```python
from build123d import *

# Parameters (mm, degrees)
SKETCH1_W           = 40
SKETCH1_H           = 40
BOSS_EXTRUDE1_DEPTH = 3
SKETCH3_W           = 20
SKETCH3_H           = 3
EXTRUDE_THIN1_DEPTH = 20
SKETCH4_W           = 10
SKETCH4_H           = 17
BOSS_EXTRUDE2_DEPTH = 2
EXTRUDE_THIN2_DEPTH = 20
SKETCH6_R           = 12.5
CUT_EXTRUDE1_DEPTH  = 57.789083458
SKETCH7_R           = 1.75
CUT_EXTRUDE2_DEPTH  = 55.990908339
CIRPATTERN1_COUNT   = 5
SKETCH8_R           = 1.75
CUT_EXTRUDE3_DEPTH  = 10
SKETCH9_R           = 1.75
CUT_EXTRUDE4_DEPTH  = 10
CUT_EXTRUDE5_DEPTH  = 59.72818744
FILLET1_R           = 2
FILLET3_R           = 2
FILLET4_R           = 2
FILLET5_R           = 2
FILLET2_R           = 1


with BuildPart() as part:
    # Sketch1 → Boss-Extrude1 (new body)
    with BuildSketch(Plane.XY):
        with Locations((0, 20)):
            Rectangle(SKETCH1_W, SKETCH1_H)
    extrude(amount=-BOSS_EXTRUDE1_DEPTH)

    # Sketch3 → Extrude-Thin1 (add, symmetric)
    with BuildSketch(Plane(origin=(0, 0, 0), x_dir=(0, 0, -1), z_dir=(1, 0, 0))):
        with Locations((-7, -1.5)):
            Rectangle(SKETCH3_W, SKETCH3_H)
    extrude(amount=EXTRUDE_THIN1_DEPTH, both=True)

    # Sketch4 → Boss-Extrude2 (add)
    with BuildSketch(Plane(origin=(0, 0, 0), x_dir=(1, 0, 0), z_dir=(0, 1, 0))):
        with Locations((0, -8.5)):
            Rectangle(SKETCH4_W, SKETCH4_H)
    extrude(amount=BOSS_EXTRUDE2_DEPTH)

    # Sketch5 → Extrude-Thin2 (add, symmetric)
    with BuildSketch(Plane(origin=(0, 0, 0), x_dir=(0, 0, -1), z_dir=(1, 0, 0))):
        Polygon((-17, 17), (-17, -8), (-32, -8), (-32, -3), (-29, -3), (-29, -5), (-20, -5), (-20, 17), align=None)
    extrude(amount=EXTRUDE_THIN2_DEPTH, both=True)

    # Sketch6 → Cut-Extrude1 (cut, through all)
    with BuildSketch(Plane.XY.offset(32)):
        with Locations((0, 20)):
            Circle(SKETCH6_R)
    extrude(amount=-CUT_EXTRUDE1_DEPTH, mode=Mode.SUBTRACT)

    # Sketch7 → Cut-Extrude2 (cut, through all)
    with BuildSketch(Plane.XY):
        with Locations((0, 37.5)):
            Circle(SKETCH7_R)
    cut_extrude2 = extrude(amount=-CUT_EXTRUDE2_DEPTH, mode=Mode.SUBTRACT)

    # CirPattern1: Cut-Extrude2 ×5 about axis
    cirpattern1_axis = Axis((0, 20, 0), (0, 0, 1))
    for i in range(1, CIRPATTERN1_COUNT):
        add(cut_extrude2.rotate(cirpattern1_axis, i * 360 / CIRPATTERN1_COUNT), mode=Mode.SUBTRACT)

    # Sketch8 → Cut-Extrude3 (cut)
    with BuildSketch(Plane.XY.offset(20)):
        with Locations(Location((10.286241915, 5.842202598, 0), (0, 0, 216))):
            Circle(SKETCH8_R)
    extrude(amount=-CUT_EXTRUDE3_DEPTH, mode=Mode.SUBTRACT)

    # Sketch9 → Cut-Extrude4 (cut)
    with BuildSketch(Plane.XY.offset(20)):
        with Locations(Location((-10.286241915, 5.842202598, 0), (0, 0, 144))):
            Circle(SKETCH9_R)
    extrude(amount=-CUT_EXTRUDE4_DEPTH, mode=Mode.SUBTRACT)

    # Sketch10 → Cut-Extrude5 (cut, through all)
    with BuildSketch(Plane(origin=(0, -5, 0), x_dir=(1, 0, 0), z_dir=(0, 1, 0))):
        with BuildLine():
            Line((-10, -22), (10, -22))
            ThreePointArc((10, -22), (12.5, -24.5), (10, -27))
            Line((10, -27), (-10, -27))
            ThreePointArc((-10, -27), (-12.5, -24.5), (-10, -22))
        make_face()
    extrude(amount=-CUT_EXTRUDE5_DEPTH, mode=Mode.SUBTRACT)

    # Fillet1
    fillet1_edges = [part.edges().sort_by_distance(p)[0] for p in [
        (5, 0, 8.5),
    ]]
    fillet(fillet1_edges, radius=FILLET1_R - 0.0001)  # a hair under: the kernel refuses the full size

    # Fillet3
    fillet3_edges = [part.edges().sort_by_distance(p)[0] for p in [
        (5, 2, 8.5),
    ]]
    fillet(fillet3_edges, radius=FILLET3_R)

    # Fillet4
    fillet4_edges = [part.edges().sort_by_distance(p)[0] for p in [
        (-5, 2, 8.5),
    ]]
    fillet(fillet4_edges, radius=FILLET4_R - 0.0001)  # a hair under: the kernel refuses the full size

    # Fillet5
    fillet5_edges = [part.edges().sort_by_distance(p)[0] for p in [
        (-5, 0, 8.5),
    ]]
    fillet(fillet5_edges, radius=FILLET5_R)

    # Fillet2
    fillet2_edges = [part.edges().sort_by_distance(p)[0] for p in [
        (13.49995, 0, 0),
        (5.9999375, 0.267943012, 17),
        (0.26787806, 2, 0),
        (5.9999375, 0.267943012, 0),
        (4.535868621, 1.73204359, 0),
        (4.535868621, 1.73204359, 17),
        (0.26787806, 2, 17),
        (-4.0000625, 1.732056988, 17),
        (-4.0000625, 1.732056988, 0),
        (-13.23207194, 0, 17),
        (-5.464131379, 0.26795641, 17),
        (-5.464131379, 0.26795641, 0),
        (13.49995, 0, 17),
        (-13.23207194, 0, 0),
    ]]
    fillet(fillet2_edges, radius=FILLET2_R)


solid = part.part
```
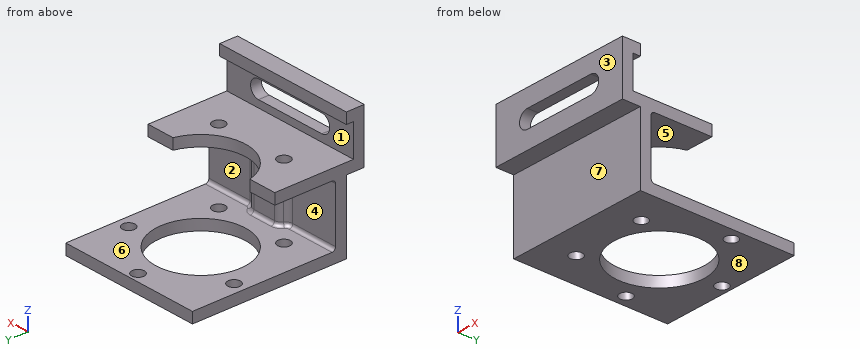
Source: CAD feature listing. Evaluate the final solid. Frame: model axes, mm. Face numbers are marked on the shaded views. A direction names the side the tool comes from. Give positions to 0.01 mm unless a question says otherwise; leave off trailing zeros. Loops run counter-clockwise (first coordinate to the right, second up) from the corner with the lowest first, then second, coordinate; pieces in that order, holes last. Notation, with made-up numbers: (-2, -2) -> (41, -2) arc R35 cw to (41, 36) -> close; hole circle Ø8 at (56, 27). An arc over 180 degrees is marked (long way). Put each result on its own line as item: value. Start each with the question number.
1) Material intervals for probe 1 along Y at (x, z) = (0, -2); probe 2 along Z at (x, y) = (-5.5, 8.5); probe 3 along Y at (x, z) = (14, 10.5), sorted ascending.
2) Contact query for flat-ended pins moving along their axis: P1, Ø6, axis at x = -14.5, z = 9.5, coming from the -Y side; P2, Ø15, axis at x = 0, y = 20, coming from the +Z side; P3, Ø1.5, axis at x = -15, z = 18, coming from the +Y side; P4, Ø12, axis at x = -10.5, y = 3.5, coming from the +Z side. Output: stop coordinate, or through.
3) Cut plane C-C (x = 0). Return loops of the section in (y, z).
4) Reachability of the marked faces 1, 2, 3 and 4 from +Z, -Z, +X, -X, +Y, -Y: full face, straight path, thin tool, end or side. Return the list, or none.
5) Draft query along Z for the marked faces 5, 6, 7 and 8. Return one class per face: released by +Z, released by -Z, zero draft, split by the parting line, or undercut.
6) Cut plane B-B (y = 20). Return loops of the section in (x, z), then the cut area to 3 significant figures.
7) Cut plane A-A (z = 26). Return loops of the section in (x, y).
Results are:
1. probe 1: y = -3 to 7.5, 32.5 to 35.75, 39.25 to 40
1. probe 2: z = -3 to 0, 17 to 20
1. probe 3: y = -3 to 0
2. P1: stops at y = -3
2. P2: passes through
2. P3: stops at y = 17
2. P4: stops at z = 20
3. outline: (-8, 17) -> (-3, 17) -> (-3, -3) -> (7.5, -3) -> (7.5, 0) -> (3, 0) arc R1 cw to (2, 1) -> (2, 16) arc R1 cw to (3, 17) -> (7.5, 17) -> (7.5, 20) -> (-5, 20) -> (-5, 22) -> (-8, 22) -> close; (-8, 27) -> (-5, 27) -> (-5, 29) -> (-3, 29) -> (-3, 32) -> (-8, 32) -> close; (32.5, -3) -> (35.75, -3) -> (35.75, 0) -> (32.5, 0) -> close; (39.25, -3) -> (40, -3) -> (40, 0) -> (39.25, 0) -> close
4. face 1: +X, -X, +Y
4. face 2: +X, +Y
4. face 3: +Z, -Z, +X, -X, -Y
4. face 4: -X, +Y
5. face 5: undercut
5. face 6: undercut
5. face 7: zero draft
5. face 8: released by -Z
6. outline: (-20, -3) -> (-12.5, -3) -> (-12.5, 0) -> (-20, 0) -> close; (12.5, -3) -> (20, -3) -> (20, 0) -> (12.5, 0) -> close
6. area: 45.0 mm2
7. outline: (-20, -8) -> (-12, -8) -> (-12, -5) -> (-20, -5) -> close; (12, -8) -> (20, -8) -> (20, -5) -> (12, -5) -> close
